from build123d import *

# Parameters (mm, degrees)
SKETCH1_R           = 28
BOSS_EXTRUDE1_DEPTH = 6
SKETCH2_R           = 19
BOSS_EXTRUDE2_DEPTH = 0.5
SKETCH3_R           = 17.5
BOSS_EXTRUDE3_DEPTH = 6.5
SKETCH4_R           = 1.05
CUT_EXTRUDE1_DEPTH  = 3
CIRPATTERN1_COUNT   = 6
SKETCH5_R           = 11.5
CUT_EXTRUDE2_DEPTH  = 3.5
SKETCH6_R           = 10
CUT_EXTRUDE3_DEPTH  = 9.5
SKETCH7_R           = 1.6
CUT_EXTRUDE4_DEPTH  = 13
CUT_EXTRUDE10_DEPTH = 5
CHAMFER1_SIZE       = 1
SKETCH13_R          = 1.6
BOSS_EXTRUDE4_DEPTH = 6
SKETCH14_R          = 2
CUT_EXTRUDE12_DEPTH = 4
CIRPATTERN3_COUNT   = 4
SKETCH15_R          = 22.5
CUT_EXTRUDE13_DEPTH = 3.5
BOSS_EXTRUDE5_START = 2
SKETCH16_R          = 1.75
SKETCH16_R_2        = 1.05
BOSS_EXTRUDE5_DEPTH = 2
CIRPATTERN4_COUNT   = 6
CHAMFER2_SIZE       = 0.7
CHAMFER3_SIZE       = 0.7
CHAMFER4_SIZE       = 1
CIRPATTERN5_COUNT   = 6


with BuildPart() as part:
    # Sketch1 → Boss-Extrude1 (new body)
    with BuildSketch(Plane(origin=(0, 0, 0), x_dir=(1, 0, 0), z_dir=(0, 1, 0))):
        with Locations(Location((0, 0, 0), (0, 0, 270))):
            Circle(SKETCH1_R)
    extrude(amount=BOSS_EXTRUDE1_DEPTH)

    # Sketch2 → Boss-Extrude2 (add)
    with BuildSketch(Plane(origin=(0, 6, 0), x_dir=(1, 0, 0), z_dir=(0, 1, 0))):
        with Locations(Location((0, 0, 0), (0, 0, 270))):
            Circle(SKETCH2_R)
    extrude(amount=BOSS_EXTRUDE2_DEPTH)

    # Sketch3 → Boss-Extrude3 (add)
    with BuildSketch(Plane(origin=(0, 6.5, 0), x_dir=(1, 0, 0), z_dir=(0, 1, 0))):
        with Locations(Location((0, 0, 0), (0, 0, 90))):
            Circle(SKETCH3_R)
    extrude(amount=BOSS_EXTRUDE3_DEPTH)

    # Sketch4 → Cut-Extrude1 (cut)
    with BuildSketch(Plane(origin=(0, 13, 0), x_dir=(1, 0, 0), z_dir=(0, 1, 0))):
        with Locations(Location((0, 15.5, 0), (0, 0, 270))):
            Circle(SKETCH4_R)
    cut_extrude1 = extrude(amount=-CUT_EXTRUDE1_DEPTH, mode=Mode.SUBTRACT)

    # CirPattern1: Cut-Extrude1 ×6 about axis
    cirpattern1_axis = Axis((0, 0, 0), (0, 1, 0))
    for i in range(1, CIRPATTERN1_COUNT):
        add(cut_extrude1.rotate(cirpattern1_axis, i * 360 / CIRPATTERN1_COUNT), mode=Mode.SUBTRACT)

    # Sketch5 → Cut-Extrude2 (cut)
    with BuildSketch(Plane(origin=(0, 13, 0), x_dir=(1, 0, 0), z_dir=(0, 1, 0))):
        with Locations(Location((0, 0, 0), (0, 0, 270))):
            Circle(SKETCH5_R)
    extrude(amount=-CUT_EXTRUDE2_DEPTH, mode=Mode.SUBTRACT)

    # Sketch6 → Cut-Extrude3 (cut)
    with BuildSketch(Plane(origin=(0, 9.5, 0), x_dir=(1, 0, 0), z_dir=(0, 1, 0))):
        with Locations(Location((0, 0, 0), (0, 0, 270))):
            Circle(SKETCH6_R)
    extrude(amount=-CUT_EXTRUDE3_DEPTH, mode=Mode.SUBTRACT)

    # Sketch7 → Cut-Extrude4 (cut)
    with BuildSketch(Plane(origin=(0, 13, 0), x_dir=(1, 0, 0), z_dir=(0, 1, 0))):
        with Locations(Location((7.5, 12.990381057, 0), (0, 0, 270))):
            Circle(SKETCH7_R)
    cut_extrude4 = extrude(amount=-CUT_EXTRUDE4_DEPTH, mode=Mode.SUBTRACT)

    # Sketch9 → Cut-Extrude10 (cut)
    with BuildSketch(Plane.XZ):
        Polygon((7.5, -9.641749495), (4.6, -11.316065276), (4.6, -14.664696837), (7.5, -16.339012618), (10.4, -14.664696837), (10.4, -11.316065276), align=None)
    cut_extrude10 = extrude(amount=-CUT_EXTRUDE10_DEPTH, mode=Mode.SUBTRACT)

    # Chamfer1
    chamfer1_edges = [part.edges().sort_by_distance(p)[0] for p in [
        (0, 0, -10),
    ]]
    chamfer(chamfer1_edges, length=CHAMFER1_SIZE)

    # Sketch13 → Boss-Extrude4 (add)
    with BuildSketch(Plane(origin=(0, 6, 0), x_dir=(1, 0, 0), z_dir=(0, 1, 0))):
        with BuildLine():
            Line((4.772059529, 31.332530186), (3.027664457, 24.822359149))
            Line((3.027664457, 24.822359149), (9.789145241, 23.010625833))
            Line((9.789145241, 23.010625833), (11.533540313, 29.52079687))
            ThreePointArc((11.533540313, 29.52079687), (9.058666579, 33.80740392), (4.772059529, 31.332530186))
        make_face()
        with Locations(Location((8.152799921, 30.426663528, 0), (0, 0, 270))):
            Circle(SKETCH13_R, mode=Mode.SUBTRACT)
    boss_extrude4 = extrude(amount=-BOSS_EXTRUDE4_DEPTH)

    # Sketch14 → Cut-Extrude12 (cut)
    with BuildSketch(Plane(origin=(0, 6, 0), x_dir=(1, 0, 0), z_dir=(0, 1, 0))):
        with Locations(Location((8.152799921, 30.426663528, 0), (0, 0, 270))):
            Circle(SKETCH14_R)
    cut_extrude12 = extrude(amount=-CUT_EXTRUDE12_DEPTH, mode=Mode.SUBTRACT)

    # CirPattern3: Boss-Extrude4, Cut-Extrude12 ×4 about axis
    cirpattern3_axis = Axis((0, 0, 0), (0, 1, 0))
    add([boss_extrude4.rotate(cirpattern3_axis, i * 360 / CIRPATTERN3_COUNT) for i in range(1, CIRPATTERN3_COUNT)])
    add([cut_extrude12.rotate(cirpattern3_axis, i * 360 / CIRPATTERN3_COUNT) for i in range(1, CIRPATTERN3_COUNT)], mode=Mode.SUBTRACT)

    # Sketch15 → Cut-Extrude13 (cut)
    with BuildSketch(Plane.XZ):
        with Locations(Location((0, 0, 0), (0, 0, 270))):
            Circle(SKETCH15_R)
    extrude(amount=-CUT_EXTRUDE13_DEPTH, mode=Mode.SUBTRACT)

    # Sketch16 → Boss-Extrude5 (add)
    with BuildSketch(Plane(origin=(0, 13, 0), x_dir=(1, 0, 0), z_dir=(0, 1, 0)).offset(BOSS_EXTRUDE5_START)):
        with Locations(Location((0, 15.5, 0), (0, 0, 270))):
            Circle(SKETCH16_R)
        with Locations(Location((0, 15.5, 0), (0, 0, 270))):
            Circle(SKETCH16_R_2, mode=Mode.SUBTRACT)
    boss_extrude5 = extrude(amount=-BOSS_EXTRUDE5_DEPTH)

    # CirPattern4: Boss-Extrude5 ×6 about axis
    cirpattern4_axis = Axis((0, 0, 0), (0, 1, 0))
    for i in range(1, CIRPATTERN4_COUNT):
        add(boss_extrude5.rotate(cirpattern4_axis, i * 360 / CIRPATTERN4_COUNT))

    # Chamfer2
    # the kernel refuses this chamfer: 0.7 mm, written as the material it takes off along each edge
    with BuildSketch(Plane(origin=(0, 13, 0), x_dir=(0, 0, -1), z_dir=(1, 0, 0))) as chamfer2_piece_1_section:
        Polygon((17.5, -CHAMFER2_SIZE), (17.5 - CHAMFER2_SIZE, 0), (17.5, 0), align=None)
    chamfer2_piece_1 = revolve(axis=Axis((0, 13, 0), (0, 1, 0)), mode=Mode.PRIVATE)
    chamfer2_piece_1 = chamfer2_piece_1 - Plane(origin=(-13.423393759, 12.425021075, 7.75), x_dir=(0.8660254037844388, 0, -0.4999999999999996), z_dir=(0, 1, 0)) * Cylinder(1.75, 71, mode=Mode.PRIVATE)
    chamfer2_piece_1 = chamfer2_piece_1 - Plane(origin=(0, 12.425021075, 15.5), x_dir=(0, 0, -1), z_dir=(0, 1, 0)) * Cylinder(1.75, 71, mode=Mode.PRIVATE)
    chamfer2_piece_1 = chamfer2_piece_1 - Plane(origin=(13.423393759, 12.425021075, 7.75), x_dir=(-0.8660254037844384, 0, -0.5000000000000007), z_dir=(0, 1, 0)) * Cylinder(1.75, 71, mode=Mode.PRIVATE)
    chamfer2_piece_1 = chamfer2_piece_1 - Plane(origin=(-13.423393759, 12.425021075, -7.75), x_dir=(0.8660254037844386, 0, 0.5000000000000003), z_dir=(0, 1, 0)) * Cylinder(1.75, 71, mode=Mode.PRIVATE)
    chamfer2_piece_1 = chamfer2_piece_1 - Plane(origin=(0, 12.425021075, -15.5), x_dir=(0, 0, 1), z_dir=(0, 1, 0)) * Cylinder(1.75, 71, mode=Mode.PRIVATE)
    chamfer2_piece_1 = chamfer2_piece_1 - Plane(origin=(13.423393759, 12.425021075, -7.75), x_dir=(-0.8660254037844387, 0, 0.49999999999999994), z_dir=(0, 1, 0)) * Cylinder(1.75, 71, mode=Mode.PRIVATE)
    add(chamfer2_piece_1, mode=Mode.SUBTRACT)

    # Chamfer3
    chamfer3_edges = [part.edges().sort_by_distance(p)[0] for p in [
        (0, 13, -11.5),
    ]]
    chamfer(chamfer3_edges, length=CHAMFER3_SIZE)

    # Chamfer4
    chamfer4_edges = [part.edges().sort_by_distance(p)[0] for p in [
        (0, 0, 22.5),
        (0, 3.5, 22.5),
    ]]
    chamfer(chamfer4_edges, length=CHAMFER4_SIZE)

    # CirPattern5: Cut-Extrude4, Cut-Extrude10 ×6 about axis
    cirpattern5_axis = Axis((0, 0, 0), (0, 1, 0))
    add([cut_extrude4.rotate(cirpattern5_axis, i * 360 / CIRPATTERN5_COUNT) for i in range(1, CIRPATTERN5_COUNT)], mode=Mode.SUBTRACT)
    add([cut_extrude10.rotate(cirpattern5_axis, i * 360 / CIRPATTERN5_COUNT) for i in range(1, CIRPATTERN5_COUNT)], mode=Mode.SUBTRACT)


solid = part.part
For this review, take the finished solid that the model builds, in its own axes (mm). A direction names the side the tool comes from. Give positions to 0.01 mm unless a question says otherwise; leave off trailing zeros. Answer in a Markdown table with one row per item. Add a question column.
(1) Consider section A-A on z = 0. Give the number of separate pieces and of enclosed holes in the cut face, and give its area (3 significant figures).
(2) For faces 4 (the face through (-6.07, 4.24, 10.467)), 5 (the face through (-8.241, 4.028, 32.425)), 6 (the face through (16.56, 9.06, 0.35)), list the 3-axis set-ups (+Z, -Z, +X, -X, +Y, -Y) from which the entire face can be reached by the end or side of a thin tool; tool diameter is ignored.
(3) Wall thickness on probe 1 along Z at (x, y) = (-7.5, 9); probe 2 along X at (y, z) = (11.55, -7.75); probe 3 along X at (y, z) = (1.75, 9): over which ranges is each line inside the solid? List them lowest first. Write a range as [from, to].
(4) For pin 1 (1.6 mm diameter, centred on y = 4.5, z = -0.5, fed in from -X); pin 2 (2.5 mm diameter, centred on x = 13.42, z = -7.75, fed in from -Y); pin 3 (4 mm diameter, centred on x = 18, y = 4, fed in from +Z), all flat-tipped, find the tip position at first contact; note any pin that passes through.
(5) Mouldability with a two-part tool opening along Z and no side actions: class faces 1 (the face through (-33.787, 3.042, -9.133)), 2 (the face through (-6.07, 4.24, -15.514)), 3 (the face through (-20, 0, 13)) as +Z half, -Z half, draft (parallel to the pull), parting line (faces both ways), or undercut.
Evaluation:
| question | item | result |
|---|---|---|
| 1 | separate pieces | 4 |
| 1 | enclosed holes | 0 |
| 1 | area | 155 mm^2 |
| 2 | face 4 | -Y |
| 2 | face 5 | +Y |
| 2 | face 6 | +Y, -Y |
| 3 | probe 1 | z = [-15.81, -14.59], [-11.39, -6.61], [6.61, 11.39], [14.59, 15.81] |
| 3 | probe 2 | x = [-15.69, -14.47], [-12.37, -8.5], [8.5, 12.37], [14.47, 15.69] |
| 3 | probe 3 | x = [-26.51, -20.62], [20.62, 29.07], [31.78, 33.82] |
| 4 | pin 1 | stops at x = -28 |
| 4 | pin 2 | stops at y = 3.5 |
| 4 | pin 3 | stops at z = 22.98 |
| 5 | face 1 | parting line |
| 5 | face 2 | undercut |
| 5 | face 3 | draft |
